Can you work these out from the model? Positions are in its coordinate system, mm. Give positions to 0.01 mm unless a question says otherwise; leave off trailing zeros. Write each loop counter-clockwise with the first axis right and the second up, starting at its lowest first coordinate (ties: lowest second). Pieces come first, ordered by that corner, then holes. Notation, with made-up numbers: (45.25, -38) -> (57.25, -38) arc R18 cw to (57.25, -11) -> close; hole circle Ø10 at (7.5, 65.25). An arc over 180 degrees is marked (long way). One line per item, written item: value.
from build123d import *

# Parameters (mm, degrees)
SKETCH3_R          = 3
CUT_EXTRUDE5_DEPTH = 10
CIRPATTERN2_COUNT  = 15
SKETCH4_R          = 3
SKETCH4_R_2        = 2
CUT_EXTRUDE7_DEPTH = 10
CIRPATTERN3_COUNT  = 15


with BuildPart() as part:
    # Sketch1 → Revolve1 (revolve)
    with BuildSketch(Plane.XY):
        Polygon((90, 80), (50, 0), (0, 0), (0, 5), (5, 5), (46.909830056, 5), (81.909830056, 75), (84.409830056, 80), align=None)
    revolve(axis=Axis((0, 0, 0), (0, 1, 0)))

    # Sketch3 → Cut-Extrude5 (cut)
    with BuildSketch(Plane(origin=(0, 5, 0), x_dir=(1, 0, 0), z_dir=(0, 1, 0))):
        with Locations((0, 40)):
            Circle(SKETCH3_R)
    cut_extrude5 = extrude(amount=-CUT_EXTRUDE5_DEPTH, mode=Mode.SUBTRACT)

    # CirPattern2: Cut-Extrude5 ×15 about axis
    cirpattern2_axis = Axis((0, 0, 0), (0, 1, 0))
    for i in range(1, CIRPATTERN2_COUNT):
        add(cut_extrude5.rotate(cirpattern2_axis, i * 360 / CIRPATTERN2_COUNT), mode=Mode.SUBTRACT)

    # Sketch4 → Cut-Extrude7 (cut)
    with BuildSketch(Plane(origin=(0, 5, 0), x_dir=(1, 0, 0), z_dir=(0, 1, 0))):
        with Locations((0, 30)):
            Circle(SKETCH4_R)
        with Locations((0, 20)):
            Circle(SKETCH4_R)
        Circle(SKETCH4_R_2)
        with Locations((0, 10)):
            Circle(SKETCH4_R_2)
    cut_extrude7 = extrude(amount=-CUT_EXTRUDE7_DEPTH, mode=Mode.SUBTRACT)

    # CirPattern3: Cut-Extrude7 ×15 about axis
    cirpattern3_axis = Axis((0, 0, 0), (0, 1, 0))
    for i in range(1, CIRPATTERN3_COUNT):
        add(cut_extrude7.rotate(cirpattern3_axis, i * 360 / CIRPATTERN3_COUNT), mode=Mode.SUBTRACT)


solid = part.part
1) If we section it at B-B (y = 47): Write out the boundary of the cut face in (x, z).
Answer list:
outline: circle Ø147 at (0, 0); hole circle Ø135.82 at (0, 0)
2) I need wall thicknesses on L1, parallel to Z at x = 0, y = 4; L2, parallel to Z at x = 48, y = 55; L3, parallel to Z at x = -25, y = 55. Which ranges of each line are inside material? Lowest first, please.
Answer list:
L1: z = -52 to -43, -37 to -33, -27 to -23, -17 to -12, -8 to -2, 2 to 52
L2: z = -60.85 to -53.54, 53.54 to 60.85
L3: z = -73.36 to -67.42, 67.42 to 73.36
3) If we section it at A-A (y = 13): Write out the boundary of the cut face in (x, z), and give its area (3 significant figures).
Answer list:
outline: circle Ø113 at (0, 0); hole circle Ø101.82 at (0, 0)
area: 1,890 mm^2
4) Will these pins go through, and if not, where does the flat tip stop? pin 1 (2.5 mm diameter, centred on x = -4.07, z = -9.14, fed in from +Y); pin 2 (3 mm diameter, centred on y = 51, z = -7, fed in from +X); pin 3 (9.5 mm diameter, centred on x = 0, z = -30, fed in from +Y); pin 4 (4 mm diameter, centred on y = 70.5, z = -51.5, fed in from -X).
Answer list:
pin 1: passes through
pin 2: stops at x = 75.94
pin 3: stops at y = 5
pin 4: stops at x = -69.86
